The figure shows three views and two pictorial views of one solid part (mm, origin at its lowest corner). Answer the questions. Round coordinates to 2 decimals unless told otherwise and drop trailing zeros. Write each loop counter-clockwise with the first axis right and the second up, starting at its lowest first coordinate (ties: lowest second). Pieces come first, ordered by that corner, then holes. Notation, with made-up numbers: (42.25, 56) -> (87.25, 56) arc R18 ccw to (87.25, 84) -> close; hole circle Ø5 at (-33, 22.25). An arc over 180 degrees is marked (long way). One line per item, written item: value.
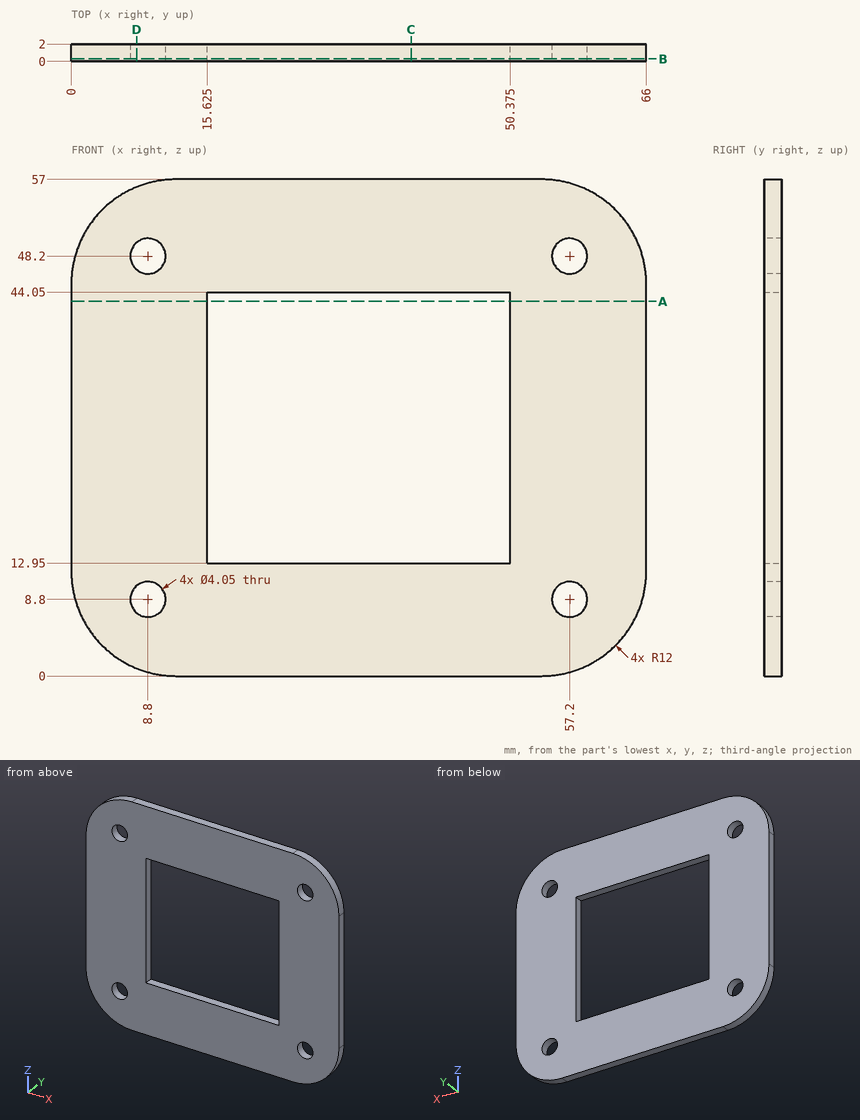
(1) Find section B-B on y = 0.3. Give the vertices of the cut face in (x, z) (3 decimals), plus the area to 3 significant figures.
Reported:
outline: (0, 12) arc R12 ccw to (12, 0) -> (54, 0) arc R12 ccw to (66, 12) -> (66, 45) arc R12 ccw to (54, 57) -> (12, 57) arc R12 ccw to (0, 45) -> close; hole circle Ø4.05 at (8.8, 8.8); hole circle Ø4.05 at (8.8, 48.2); hole (15.625, 12.95) -> (50.375, 12.95) -> (50.375, 44.05) -> (15.625, 44.05) -> close; hole circle Ø4.05 at (57.2, 8.8); hole circle Ø4.05 at (57.2, 48.2)
area: 2,510 mm2
(2) Find section A-A on z = 43. Give the vertices of the cut face in (x, y) (3 decimals), plus the area to 3 significant figures.
Reported:
outline: (0, 0) -> (15.625, 0) -> (15.625, 2) -> (0, 2) -> close; (50.375, 0) -> (66, 0) -> (66, 2) -> (50.375, 2) -> close
area: 62.5 mm2
(3) Find section C-C on x = 39. Give the vertices of the cut face in (y, z).
Reported:
outline: (0, 0) -> (2, 0) -> (2, 12.95) -> (0, 12.95) -> close; (0, 44.05) -> (2, 44.05) -> (2, 57) -> (0, 57) -> close
(4) Find section D-D on x = 7.5. Give the vertices of the cut face in (y, z).
Reported:
outline: (0, 0.88) -> (2, 0.88) -> (2, 7.25) -> (0, 7.25) -> close; (0, 10.35) -> (2, 10.35) -> (2, 46.65) -> (0, 46.65) -> close; (0, 49.75) -> (2, 49.75) -> (2, 56.12) -> (0, 56.12) -> close
(5) Consider probe 1 along Z at (x, y) = (39, 0.9); probe 2 along X at (y, z) = (1.05, 27) (3 decimals); probe 3 along X at (y, z) = (0.6, 49). Determine where each line is inside the solid, lowest interval first.
Reported:
probe 1: z = 0 to 12.95, 44.05 to 57
probe 2: x = 0 to 15.625, 50.375 to 66
probe 3: x = 0.69 to 6.94, 10.66 to 55.34, 59.06 to 65.31
